Answer from the drawing. Dimensions are ordinates in mm from the lowest x, y and z of the part. A direction names the side the tool comes from. Give positions to 0.01 mm unless a question says otherwise; leave off trailing zeros. Loops run counter-clockwise (first coordinate to the right, second up) from the corner with the lowest first, then second, coordinate; pieces in that order, holes last.
Item 1: Section C-C, the plane z = 3.2 is taken. Give the vertices of the cut face in (x, y).
Item 2: The mould has two halves that part along Y. Classify the marked faces 1, 2 and 3: pulls with the +Y half, pulls with the -Y half, needs draft (parallel to the pull), parting line crosses it, or undercut.
Item 3: Consider line 1 along X through (y, z) = (3.5, 0.5); line 2 along X through (y, z) = (25.5, 3.25); line 3 along Y through (x, z) = (4, 0.4). Determine where each line is inside the solid, lowest interval first.
Item 4: Each of these flat-tipped pins is pushed along its axis until it touches: pin 1 Ø3 at (x, y) = (32, 17) entering from -Z; pin 2 Ø2 at (x, y) = (13.5, 26) entering from +Z; pin 3 Ø1.6 at (y, z) = (1, 3.5) entering from -X; pin 4 Ø0.6 at (x, z) = (32.5, 1) entering from -Y. Where does it stop, or does it pass through?
Item 5: A tool of negligible diameter and unlimited length cuts with its end or side. For the marked faces 4, 5 and 6, from which of +Z, -Z, +X, -X, +Y, -Y can it reach the whole face along a straight path? Write none if from no direction.
Item 6: Section B-B, the plane x = 16 is taken. Give the vertices of the cut face in (y, z).
Item 7: Section D-D, the plane y = 12.5 is taken. Give the vertices of the cut face in (x, z).
Item 8: Section A-A, the plane y = 23.25 is taken. Give the vertices of the cut face in (x, z).
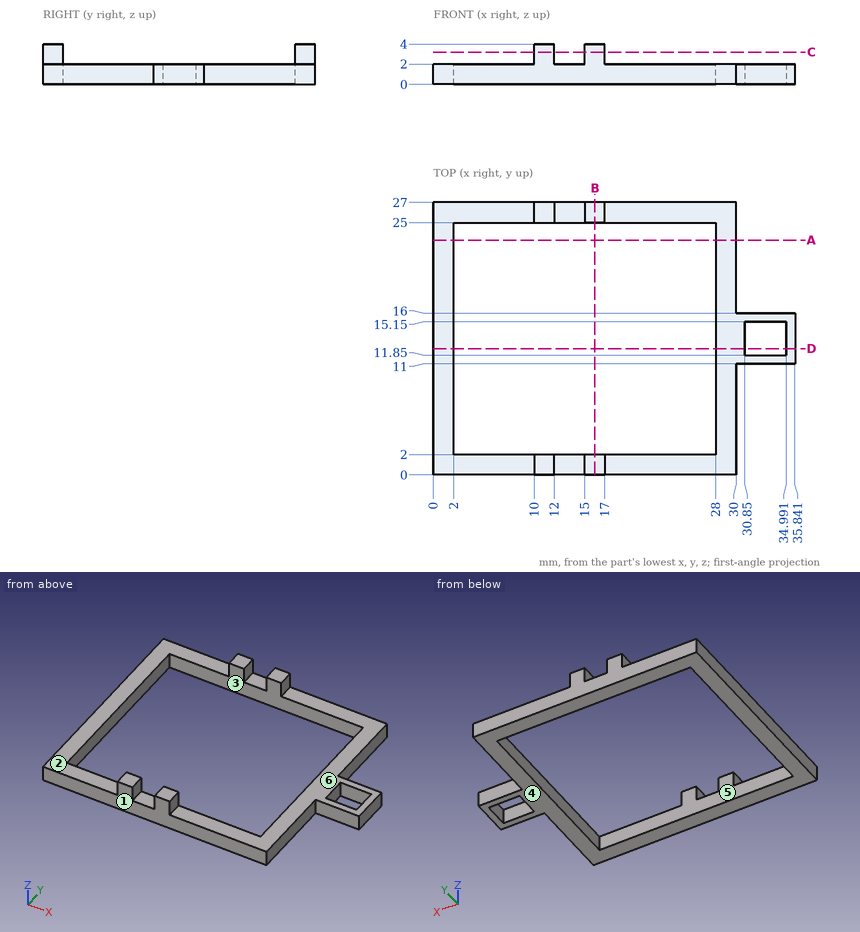
Worked answers:
1. outline: (10, 0) - (12, 0) - (12, 2) - (10, 2) - close; (10, 25) - (12, 25) - (12, 27) - (10, 27) - close; (15, 0) - (17, 0) - (17, 2) - (15, 2) - close; (15, 25) - (17, 25) - (17, 27) - (15, 27) - close
2. face 1: pulls with the -Y half
2. face 2: needs draft
2. face 3: undercut
3. line 1: x = 0 to 2, 28 to 30
3. line 2: x = 10 to 12, 15 to 17
3. line 3: y = 0 to 2, 25 to 27
4. pin 1: stops at z = 0
4. pin 2: stops at z = 2
4. pin 3: stops at x = 10
4. pin 4: stops at y = 11
5. face 4: -Z, +X, -X, +Y, -Y
5. face 5: +Z, -Z
5. face 6: +Z, +X, +Y, -Y
6. outline: (0, 0) - (2, 0) - (2, 4) - (0, 4) - close; (25, 0) - (27, 0) - (27, 4) - (25, 4) - close
7. outline: (0, 0) - (2, 0) - (2, 2) - (0, 2) - close; (28, 0) - (30.85, 0) - (30.85, 2) - (28, 2) - close; (34.99, 0) - (35.84, 0) - (35.84, 2) - (34.99, 2) - close
8. outline: (0, 0) - (2, 0) - (2, 2) - (0, 2) - close; (28, 0) - (30, 0) - (30, 2) - (28, 2) - close
